Design review of the part built by this model. Coordinates are the model's own, in mm. A direction names the side the tool comes from. Round coordinates to 2 decimals unless told otherwise and drop trailing zeros. Order: outer loops, then holes, each group sorted by start corner. A loop starts at its lowest first (then second) coordinate and runs counter-clockwise, first axis right, second up. Notation, with made-up numbers: M 52.25,7.5 L 86.25,7.5 A24 ccw 86.25,24.5 Z; hole C -30.5,34.25 d4. An arc over 180 degrees is marked long. Use a Markdown table: item, result. Add a question column.
(1) For pin 1 (3 mm diameter, centred on x = 60, z = 43, fed in from -Y); pin 2 (8 mm diameter, centred on y = -141, z = -43.5, fed in from -X); pin 3 (1 mm diameter, centred on x = 4, y = -86.5, fed in from +Z), all flat-tipped, find the tip position at first contact; note any pin that passes through.
(2) Machinability: for faces 1 (the face through (56.133, -175.07, -12.465)), 2 (the face through (51.721, -90.898, -67.453)), which of the approach directions +Z, -Z, +X, -X, +Y, -Y give a long, thin tool a straight path to every point of the face, cutting with its end or side? Answer none if there is none.
(3) Take a section at A-A (y = -85.5). Write out the cut boundary in (x, z).
(4) The part is to be moulded in two halves that separate along X. For faces 3 (the face through (-1.342, -178.125, -0.298)), 4 (the face through (-1, 0, -12)), 5 (the face through (56.133, -5.07, -12.465)), say which applies: released by +X, released by -X, zero draft, split by the parting line, or undercut.
(5) To check wall thickness, follow probe 1 along X at (y, z) = (-37, 0); probe 2 along X at (y, z) = (-18, -8); probe 3 along X at (y, z) = (-24, -21.5). State the ranges of each line that lie inside material, in increasing order. Write a range as from..to.
```python
from build123d import *

# Parameters (mm, degrees)
SKETCH2_R          = 1.25
CUT_EXTRUDE1_DEPTH = 217.448608219
CHAMFER1_SIZE      = 2


with BuildPart() as part:
    # Sketch1 → Revolve1 (revolve)
    with BuildSketch(Plane.XY, mode=Mode.PRIVATE) as revolve1_sk:
        Polygon((0, 0), (-57.5, 0), (-57.5, -10), (-85, -25.877132403), (-85, -154.122867597), (-57.5, -170), (-57.5, -180), (0, -180), align=None)
    revolve(revolve1_sk.sketch.rotate(Axis((0, 52.509012346, 0), (0, -1, 0)), 270), axis=Axis((0, 52.509012346, 0), (0, -1, 0)))

    # Sketch2 → Cut-Extrude1 (cut, through all)
    with BuildSketch(Plane(origin=(0, 0, 0), x_dir=(1, 0, 0), z_dir=(0, 1, 0))):
        with Locations(Location((0, 0, 0), (0, 0, 270))):
            Circle(SKETCH2_R)
    extrude(amount=-CUT_EXTRUDE1_DEPTH, mode=Mode.SUBTRACT)

    # Chamfer1
    chamfer1_edges = [part.edges().sort_by_distance(p)[0] for p in [
        (0, -180, -1.25),
    ]]
    chamfer(chamfer1_edges, length=CHAMFER1_SIZE)


solid = part.part
```
Verdict:
| question | item | result |
|---|---|---|
| 1 | pin 1 | stops at y = -161.45 |
| 1 | pin 2 | stops at x = -75.26 |
| 1 | pin 3 | stops at z = 84.93 |
| 2 | face 1 | -Y |
| 2 | face 2 | +Y, -Y |
| 3 | outline | C 0,0 d170; hole C 0,0 d2.5 |
| 4 | face 3 | undercut |
| 4 | face 4 | zero draft |
| 4 | face 5 | split by the parting line |
| 5 | probe 1 | x = -85..-1.25, 1.25..85 |
| 5 | probe 2 | x = -70.91..70.91 |
| 5 | probe 3 | x = -78.87..78.87 |
